Work out the finished part from the listing and answer in its coordinate system (mm). A direction names the side the tool comes from. Coordinates: 2 decimals unless noted, no trailing zeros. Write each loop counter-clockwise with the first axis right and the second up, starting at its lowest first coordinate (ties: lowest second). Pieces come first, ordered by that corner, then holes. Notation, with made-up numbers: (75, 54.5) - (107, 54.5) arc R23 ccw to (107, 64.5) - close; hole circle Ø7 at (39, 65.25). An arc over 180 degrees is marked (long way). Use a Markdown table: item, result. Add a question column.
(1) Given pin 1 Ø5 at (x, y) = (-7.5, 8) entering from +Z; pin 2 Ø1.5 at (y, z) = (3, 36.5) entering from -X; pin 3 Ø6 at (x, z) = (15, 5.5) entering from -Y; pin 4 Ø3 at (y, z) = (8, -1) entering from +X, each flat-ended and moving along its own axis, determine where each tip first touches the part or whether it passes through.
(2) The part is cut by section A-A, the plane y = 5.25. Give the vertices of the cut face in (x, z), then the cut area to 3 significant figures.
(3) The part is cut by section B-B, the plane x = 0. Give the vertices of the cut face in (y, z).
(4) The part is cut by section D-D, the plane z = 25.5. Give the vertices of the cut face in (x, y), then the cut area to 3 significant figures.
(5) Find the intervals of material crossed by line 1 (X direction, y = 10.25, z = 1); line 2 (Z direction, x = 5.5, y = 9.5); line 3 (Z direction, x = -39, y = 3.5), in increasing order. Write a range as from..to.
(6) A tool of negligible diameter and unlimited length cuts with its end or side. For faces 4 (the face through (-0.37, 7.34, -7.62)), 5 (the face through (0, 7, 5.15)), 6 (the face through (0, 11, -10.15)), 7 (the face through (0, 9, 10.15)), 8 (the face through (0, 14, -7)), from which of +Z, -Z, +X, -X, +Y, -Y can it reach the whole face along a straight path? Write none if from no direction.
(7) For a pull along X with two mould halves and no side action, classify faces 1 (the face through (40.874, 1.972, -39.151)), 2 (the face through (-4, 4, -11)), 3 (the face through (-10.9, 9, 0)) as released by +X, released by -X, zero draft, split by the parting line, or undercut.
(8) The part is cut by section C-C, the plane z = -3.5. Give the vertices of the cut face in (x, y).
from build123d import *

# Parameters (mm, degrees)
SKETCH1_R                = 2
BOSS_EXTRUDE1_DEPTH      = 4
SKETCH7_W                = 21.8
SKETCH7_H                = 20.3
SKETCH7_W_2              = 11.8
SKETCH7_H_2              = 10.3
BOSS_EXTRUDE2_DEPTH      = 10
M3_CLEARANCE_HOLE1_D     = 3.4
M3_CLEARANCE_HOLE1_DEPTH = 5
SKETCH7_2_W              = 11.8
SKETCH7_2_H              = 10.3
CUT_EXTRUDE1_DEPTH       = 10


with BuildPart() as part:
    # Sketch1 → Boss-Extrude1 (new body)
    with BuildSketch(Plane(origin=(0, 0, 0), x_dir=(1, 0, 0), z_dir=(0, 1, 0))):
        with BuildLine():
            ThreePointArc((-31.406166481, 41.715615227), (-44.547727215, 44.547727215), (-41.715615227, 31.406166481))
            ThreePointArc((-41.715615227, 31.406166481), (-20, 0), (-41.715615227, -31.406166481))
            ThreePointArc((-41.715615227, -31.406166481), (-44.547727215, -44.547727215), (-31.406166481, -41.715615227))
            ThreePointArc((-31.406166481, -41.715615227), (0, -20), (31.406166481, -41.715615227))
            ThreePointArc((31.406166481, -41.715615227), (44.547727215, -44.547727215), (41.715615227, -31.406166481))
            ThreePointArc((41.715615227, -31.406166481), (20, 0), (41.715615227, 31.406166481))
            ThreePointArc((41.715615227, 31.406166481), (44.547727215, 44.547727215), (31.406166481, 41.715615227))
            ThreePointArc((31.406166481, 41.715615227), (0, 20), (-31.406166481, 41.715615227))
        make_face()
        with Locations(Location((-38.890872965, 38.890872965, 0), (0, 0, 270))):
            Circle(SKETCH1_R, mode=Mode.SUBTRACT)
        with Locations(Location((38.890872965, 38.890872965, 0), (0, 0, 270))):
            Circle(SKETCH1_R, mode=Mode.SUBTRACT)
        with Locations(Location((38.890872965, -38.890872965, 0), (0, 0, 270))):
            Circle(SKETCH1_R, mode=Mode.SUBTRACT)
        with Locations(Location((-38.890872965, -38.890872965, 0), (0, 0, 270))):
            Circle(SKETCH1_R, mode=Mode.SUBTRACT)
    extrude(amount=BOSS_EXTRUDE1_DEPTH)

    # Sketch7 → Boss-Extrude2 (add)
    with BuildSketch(Plane.XZ.offset(-4)):
        Rectangle(SKETCH7_W, SKETCH7_H)
        Rectangle(SKETCH7_W_2, SKETCH7_H_2, mode=Mode.SUBTRACT)
    extrude(amount=-BOSS_EXTRUDE2_DEPTH)

    # M3 Clearance Hole1
    with Locations(Plane(origin=(0, 9, -10.15), x_dir=(-1, 0, 0), z_dir=(0, 0, -1))):
        with Locations((0, 0)):
            Hole(M3_CLEARANCE_HOLE1_D / 2, depth=M3_CLEARANCE_HOLE1_DEPTH)

    # Sketch7<2> → Cut-Extrude1 (cut)
    with BuildSketch(Plane.XZ.offset(-4)):
        Rectangle(SKETCH7_2_W, SKETCH7_2_H)
    extrude(amount=CUT_EXTRUDE1_DEPTH, mode=Mode.SUBTRACT)


solid = part.part
Model answer:
| question | item | result |
|---|---|---|
| 1 | pin 1 | z = 10.15 |
| 1 | pin 2 | x = -46.72 |
| 1 | pin 3 | y = 0 |
| 1 | pin 4 | x = 10.9 |
| 2 | outline | (-10.9, -10.15) - (10.9, -10.15) - (10.9, 10.15) - (-10.9, 10.15) - close; hole (-5.9, -5.15) - (5.9, -5.15) - (5.9, 5.15) - (-5.9, 5.15) - close |
| 2 | area | 321 mm^2 |
| 3 | outline | (0, -20) - (4, -20) - (4, -10.15) - (7.3, -10.15) - (7.3, -5.15) - (0, -5.15) - close; (0, 5.15) - (14, 5.15) - (14, 10.15) - (4, 10.15) - (4, 20) - (0, 20) - close; (10.7, -10.15) - (14, -10.15) - (14, -5.15) - (10.7, -5.15) - close |
| 4 | outline | (-31.74, 0) - (-18.41, 0) - (-18.41, 4) - (-31.74, 4) - close; (18.41, 0) - (31.74, 0) - (31.74, 4) - (18.41, 4) - close |
| 4 | area | 107 mm^2 |
| 5 | line 1 | -10.9..-5.9, 5.9..10.9 |
| 5 | line 2 | -10.15..-5.15, 5.15..10.15 |
| 5 | line 3 | -46.89..-40.89, -36.89..-30.24, 30.24..36.89, 40.89..46.89 |
| 6 | face 4 | -Z |
| 6 | face 5 | +Y, -Y |
| 6 | face 6 | -Z, +X, -X, +Y |
| 6 | face 7 | +Z, +X, -X, +Y |
| 6 | face 8 | +Z, -Z, +X, -X, +Y |
| 7 | face 1 | undercut |
| 7 | face 2 | zero draft |
| 7 | face 3 | released by -X |
| 8 | outline | (-20.18, 0) - (-5.9, 0) - (-5.9, 14) - (-10.9, 14) - (-10.9, 4) - (-20.18, 4) - close; (5.9, 0) - (20.18, 0) - (20.18, 4) - (10.9, 4) - (10.9, 14) - (5.9, 14) - close |
